Autodesk Inventor part; units mm, degrees
ref_plane "YZ Plane" through (0, 0, 0) normal (1, 0, 0) x (0, 1, 0)
ref_plane "XZ Plane" through (0, 0, 0) normal (0, 1, 0) x (-1, 0, 0)
ref_plane "XY Plane" through (0, 0, 0) normal (0, 0, 1) x (1, 0, 0)
ref_plane "Work Plane1" through (0, 0, 0) normal (0, 0, 1) x (1, 0, 0)
sketch "Sketch1" plane through (0, 0, 0) normal (0, 0, 1) x (1, 0, 0)
  arc A0 (20.3917, -80.7036) -> (21.6617, -79.4336) centre (20.3917, -79.4336) ccw
  line L0 (21.6617, -79.4336) -> (21.6617, -76.6142)
  arc A1 (21.6617, -76.6142) -> (20.3917, -75.3442) centre (20.3917, -76.6142) ccw
  line L1 (20.3917, -75.3442) -> (-1.8333, -75.3442)
  arc A2 (-1.8333, -75.3442) -> (-3.1033, -76.6142) centre (-1.8333, -76.6142) ccw
  line L2 (-3.1033, -76.6142) -> (-3.1033, -81.3894)
  arc A3 (-4.3733, -82.6594) -> (-3.1033, -81.3894) centre (-4.3733, -81.3894) ccw
  line L3 (-4.3733, -82.6594) -> (-7.8023, -82.6594)
  arc A4 (-7.8023, -82.6594) -> (-9.0723, -83.9294) centre (-7.8023, -83.9294) ccw
  line L4 (-9.0723, -83.9294) -> (-9.0723, -88.3998)
  arc A5 (-9.0723, -88.3998) -> (-7.8023, -89.6698) centre (-7.8023, -88.3998) ccw
  line L5 (-7.8023, -89.6698) -> (-3.3319, -89.6698)
  arc A6 (-3.3319, -89.6698) -> (-2.0619, -88.3998) centre (-3.3319, -88.3998) ccw
  line L6 (-2.0619, -88.3998) -> (-2.0619, -85.5109)
  arc A7 (-0.9806, -84.255) -> (-2.0619, -85.5109) centre (-0.7919, -85.5109) ccw
  arc A8 (-0.9806, -84.255) -> (4.2373, -80.7036) centre (-2.0619, -77.0575) ccw
  line L7 (4.2373, -80.7036) -> (20.3917, -80.7036)
  arc A9 (21.6617, -2.5224) -> (20.3917, -1.2524) centre (20.3917, -2.5224) ccw
  line L8 (4.2373, -1.2524) -> (20.3917, -1.2524)
  arc A10 (4.2373, -1.2524) -> (-0.9806, 2.299) centre (-2.0619, -4.8985) ccw
  arc A11 (-2.0619, 3.5549) -> (-0.9806, 2.299) centre (-0.7919, 3.5549) ccw
  line L9 (-2.0619, 6.4438) -> (-2.0619, 3.5549)
  arc A12 (-2.0619, 6.4438) -> (-3.3319, 7.7138) centre (-3.3319, 6.4438) ccw
  line L10 (-7.8023, 7.7138) -> (-3.3319, 7.7138)
  arc A13 (-7.8023, 7.7138) -> (-9.0723, 6.4438) centre (-7.8023, 6.4438) ccw
  line L11 (-9.0723, 1.9734) -> (-9.0723, 6.4438)
  arc A14 (-9.0723, 1.9734) -> (-7.8023, 0.7034) centre (-7.8023, 1.9734) ccw
  line L12 (-4.3733, 0.7034) -> (-7.8023, 0.7034)
  arc A15 (-3.1033, -0.5666) -> (-4.3733, 0.7034) centre (-4.3733, -0.5666) ccw
  line L13 (-3.1033, -5.3418) -> (-3.1033, -0.5666)
  arc A16 (-3.1033, -5.3418) -> (-1.8333, -6.6118) centre (-1.8333, -5.3418) ccw
  line L14 (20.3917, -6.6118) -> (-1.8333, -6.6118)
  arc A17 (20.3917, -6.6118) -> (21.6617, -5.3418) centre (20.3917, -5.3418) ccw
  line L15 (21.6617, -2.5224) -> (21.6617, -5.3418)
  arc A18 (20.3917, -81.9736) -> (22.9317, -79.4336) centre (20.3917, -79.4336) ccw
  line L16 (22.9317, -79.4336) -> (22.9317, -76.6142)
  arc A19 (22.9317, -76.6142) -> (20.3917, -74.0742) centre (20.3917, -76.6142) ccw
  line L17 (20.3917, -74.0742) -> (-1.8333, -74.0742)
  arc A20 (-1.8333, -74.0742) -> (-4.3733, -76.6142) centre (-1.8333, -76.6142) ccw
  line L18 (-4.3733, -76.6142) -> (-4.3733, -81.3894)
  line L19 (-4.3733, -81.3894) -> (-7.8023, -81.3894)
  arc A21 (-7.8023, -81.3894) -> (-10.3423, -83.9294) centre (-7.8023, -83.9294) ccw
  line L20 (-10.3423, -83.9294) -> (-10.3423, -88.3998)
  arc A22 (-10.3423, -88.3998) -> (-7.8023, -90.9398) centre (-7.8023, -88.3998) ccw
  line L21 (-7.8023, -90.9398) -> (-3.3319, -90.9398)
  arc A23 (-3.3319, -90.9398) -> (-0.7919, -88.3998) centre (-3.3319, -88.3998) ccw
  line L22 (-0.7919, -88.3998) -> (-0.7919, -85.5109)
  arc A24 (-0.7919, -85.5109) -> (4.9314, -81.9736) centre (-2.0619, -77.0575) ccw
  line L23 (4.9314, -81.9736) -> (20.3917, -81.9736)
  arc A25 (-4.3733, -5.3418) -> (-1.8333, -7.8818) centre (-1.8333, -5.3418) ccw
  line L24 (-4.3733, -5.3418) -> (-4.3733, -0.5666)
  line L25 (-4.3733, -0.5666) -> (-7.8023, -0.5666)
  arc A26 (-10.3423, 1.9734) -> (-7.8023, -0.5666) centre (-7.8023, 1.9734) ccw
  line L26 (-10.3423, 1.9734) -> (-10.3423, 6.4438)
  arc A27 (-7.8023, 8.9838) -> (-10.3423, 6.4438) centre (-7.8023, 6.4438) ccw
  line L27 (-7.8023, 8.9838) -> (-3.3319, 8.9838)
  arc A28 (-0.7919, 6.4438) -> (-3.3319, 8.9838) centre (-3.3319, 6.4438) ccw
  line L28 (-0.7919, 6.4438) -> (-0.7919, 3.5549)
  arc A29 (4.9314, 0.0176) -> (-0.7919, 3.5549) centre (-2.0619, -4.8985) ccw
  line L29 (4.9314, 0.0176) -> (20.3917, 0.0176)
  arc A30 (22.9317, -2.5224) -> (20.3917, 0.0176) centre (20.3917, -2.5224) ccw
  line L30 (22.9317, -2.5224) -> (22.9317, -5.3418)
  arc A31 (20.3917, -7.8818) -> (22.9317, -5.3418) centre (20.3917, -5.3418) ccw
  line L31 (20.3917, -7.8818) -> (-1.8333, -7.8818)
  line L32 (6.2947, -102.4206) -> (6.2947, 20.4646) construction
  line L33 (26.7417, -81.9736) -> (26.7417, 0.0176)
  line L34 (-14.1523, 0.0176) -> (-14.1523, -81.9736)
  arc A32 (-14.1523, -81.9736) -> (26.7417, -81.9736) centre (6.2947, -81.9736) ccw
  arc A33 (26.7417, 0.0176) -> (-14.1523, 0.0176) centre (6.2947, 0.0176) ccw
  point P0 (0, 0)
  point P1 (6.2947, -40.978)
  dimension "d0" = 1.27
  dimension "d1" = 1.27
  dimension "d2" = 3.81
  dimension "d3" = 3.81
  dimension "d4" = 33.0962
  dimension "d5" = 33.0962
extrude "Extrusion1" add sketch "Sketch1" against normal blind 6.35 contours A32 L34 A33 L33
sketch "Sketch2" plane through (0, 0, 0) normal (0, 0, 1) x (1, 0, 0)
  line L0 (20.3917, -7.8818) -> (-1.8333, -7.8818)
  arc A0 (-4.3733, -5.3418) -> (-1.8333, -7.8818) centre (-1.8333, -5.3418) ccw
  line L1 (-4.3733, -5.3418) -> (-4.3733, -0.5666)
  line L2 (-4.3733, -0.5666) -> (-7.8023, -0.5666)
  arc A1 (-10.3423, 1.9734) -> (-7.8023, -0.5666) centre (-7.8023, 1.9734) ccw
  line L3 (-10.3423, 1.9734) -> (-10.3423, 6.4438)
  arc A2 (-7.8023, 8.9838) -> (-10.3423, 6.4438) centre (-7.8023, 6.4438) ccw
  line L4 (-7.8023, 8.9838) -> (-3.3319, 8.9838)
  arc A3 (-0.7919, 6.4438) -> (-3.3319, 8.9838) centre (-3.3319, 6.4438) ccw
  line L5 (-0.7919, 6.4438) -> (-0.7919, 3.5549)
  arc A4 (4.9314, 0.0176) -> (-0.7919, 3.5549) centre (-2.0619, -4.8985) ccw
  line L6 (4.9314, 0.0176) -> (20.3917, 0.0176)
  arc A5 (22.9317, -2.5224) -> (20.3917, 0.0176) centre (20.3917, -2.5224) ccw
  line L7 (22.9317, -2.5224) -> (22.9317, -5.3418)
  arc A6 (20.3917, -7.8818) -> (22.9317, -5.3418) centre (20.3917, -5.3418) ccw
  line L8 (22.9317, -76.6142) -> (22.9317, -79.4336)
  arc A7 (20.3917, -81.9736) -> (22.9317, -79.4336) centre (20.3917, -79.4336) ccw
  line L9 (20.3917, -81.9736) -> (4.9314, -81.9736)
  arc A8 (-0.7919, -85.5109) -> (4.9314, -81.9736) centre (-2.0619, -77.0575) ccw
  line L10 (-0.7919, -85.5109) -> (-0.7919, -88.3998)
  arc A9 (-3.3319, -90.9398) -> (-0.7919, -88.3998) centre (-3.3319, -88.3998) ccw
  line L11 (-3.3319, -90.9398) -> (-7.8023, -90.9398)
  arc A10 (-10.3423, -88.3998) -> (-7.8023, -90.9398) centre (-7.8023, -88.3998) ccw
  line L12 (-10.3423, -88.3998) -> (-10.3423, -83.9294)
  arc A11 (-7.8023, -81.3894) -> (-10.3423, -83.9294) centre (-7.8023, -83.9294) ccw
  line L13 (-7.8023, -81.3894) -> (-4.3733, -81.3894)
  line L14 (-4.3733, -81.3894) -> (-4.3733, -76.6142)
  arc A12 (-1.8333, -74.0742) -> (-4.3733, -76.6142) centre (-1.8333, -76.6142) ccw
  line L15 (-1.8333, -74.0742) -> (20.3917, -74.0742)
  arc A13 (22.9317, -76.6142) -> (20.3917, -74.0742) centre (20.3917, -76.6142) ccw
  line L16 (26.7417, -81.9736) -> (26.7417, 0.0176)
  arc A14 (26.7417, 0.0176) -> (-14.1523, 0.0176) centre (6.2947, 0.0176) ccw
  line L17 (-14.1523, 0.0176) -> (-14.1523, -81.9736)
  arc A15 (-14.1523, -81.9736) -> (26.7417, -81.9736) centre (6.2947, -81.9736) ccw
  point P0 (0, 0)
extrude "Extrusion2" add sketch "Sketch2" along normal blind 2.54 contours L0 A0 L1 L2 A1 L3 A2 L4 A3 L5 A4 L6 A5 L7 A6 | L8 A7 L9 A8 L10 A9 L11 A10 L12 A11 L13 L14 A12 L15 A13 | A15 L17 A14 L16
fillet "Fillet1" radius 3.175 8 edges at (-14.1523, -40.978, 2.54) (6.2947, -102.4206, 2.54) (26.7417, -40.978, 2.54) (6.2947, 20.4646, 2.54) (-14.1523, -40.978, -6.35) (6.2947, 20.4646, -6.35) (26.7417, -40.978, -6.35) (6.2947, -102.4206, -6.35)
equation "\"d1\" = d0"
equation "\"d3\" = d2"
properties part number "cap"
The model under review builds one solid part; all positions refer to its coordinate system, in mm. A direction names the side the tool comes from. Round coordinates to 2 decimals unless told otherwise and drop trailing zeros. Order: outer loops, then holes, each group sorted by start corner. A loop starts at its lowest first (then second) coordinate and runs counter-clockwise, first axis right, second up. Notation, with made-up numbers: (16, 30.25) - (55, 30.25) arc R23 cw to (55, 45.25) - close; hole circle Ø2 at (13, 22.25). An arc over 180 degrees is marked (long way). Use one line per item in the form item = value.
Q1. Tool access review of faces 4 (the cylindrical face through (-3.649, -7.118, -3.131)), 5 (the flat face through (6, -40, 2.54)): name each direction out of +Z, -Z, +X, -X, +Y, -Y from which nothing blocks a thin tool from reaching the whole face with its end or side.
Response values:
face_4 = -Z
face_5 = +Z, +X, -X, +Y, -Y
Q2. Add section A-A on y = -37. Give the boundary of the cut face in (x, z) (3 decimals), then the cut area to 3 significant figures.
Response values:
outline = (-14.152, -3.175) arc R3.175 ccw to (-10.977, -6.35) - (23.567, -6.35) arc R3.175 ccw to (26.742, -3.175) - (26.742, -0.635) arc R3.175 ccw to (23.567, 2.54) - (-10.977, 2.54) arc R3.175 ccw to (-14.152, -0.635) - close
area = 355 mm^2
Q3. Add section C-C on z = 1.5. Give the boundary of the cut face in (x, y), then the cut area to 3 significant figures.
Response values:
outline = (-13.33, -81.97) arc R19.62 ccw to (25.92, -81.97) - (25.92, 0.02) arc R19.62 ccw to (-13.33, 0.02) - close
area = 4,430 mm^2
Q4. Add section B-B on z = -5. Give the number of separate pieces and of enclosed holes in the cut face, then the cut area to 3 significant figures.
Response values:
separate_pieces = 1
enclosed_holes = 2
area = 3,880 mm^2
Q5. Clearance check with flat-ended pins moving along their axes: P1, Ø1, axis at x = -6, z = 0.5, coming from the -Y side; P2, Ø0.9, axis at y = 4.5, z = -2, coming from the -X side; P3, Ø2, axis at y = 4, z = -4.5, coming from the +X side; P4, Ø2.5, axis at y = -3.5, z = -3.5, coming from the -X side. State where each tip first meets the part, or that it passes through.
Response values:
P1 = -98.47
P2 = -13.75
P3 = 26.42
P4 = -14.15
Q6. To check wall thickness, follow line 1 (Y direction, x = 5.5, z = -2); line 2 (Y direction, x = 10.5, z = -2); line 3 (X direction, y = -4, z = -0.75). State the ranges of each line that lie inside material, in increasing order.
Response values:
line_1 = -102.41 to -81.97, -74.07 to -7.88, 0.02 to 20.45
line_2 = -101.98 to -81.97, -74.07 to -7.88, 0.02 to 20.03
line_3 = -14.15 to -4.37, 22.93 to 26.74
Q7. Mouldability with a two-part tool opening along Y and no side actions: class faces 1 (the cylindrical face through (6.74, 20.46, -1.89)), 2 (the cylindrical face through (-13.247, -40.404, 1.585)), 3 (the flat face through (-6, 8.984, -3)) as pulls with the +Y half, pulls with the -Y half, needs draft (parallel to the pull), parting line crosses it, or undercut.
Response values:
face_1 = pulls with the +Y half
face_2 = needs draft
face_3 = undercut
